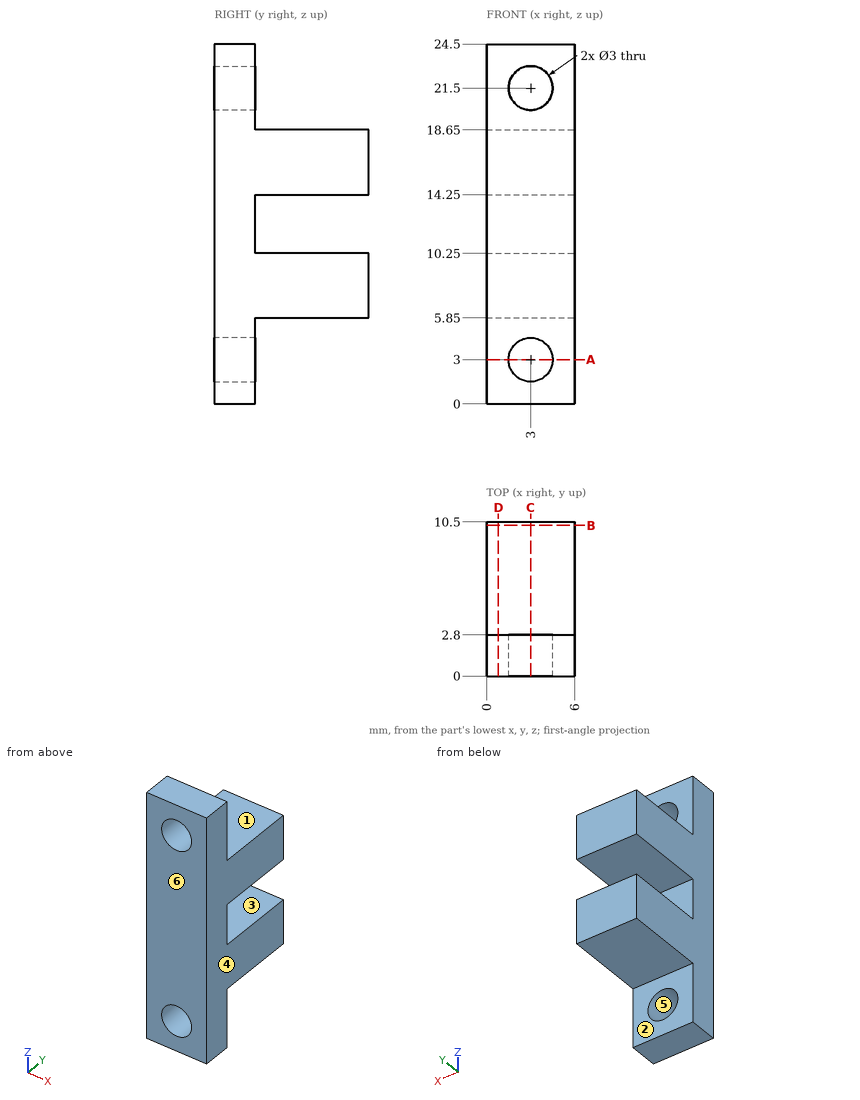
Geometry: see drawing. Coordinates: mm, zero at the bounding-box minimum. A direction names the side the tool comes from. Coordinates: 2 decimals unless noted, no trailing zeros. Order: outer loops, then holes, each group sorted by start corner. A loop starts at its lowest first (then second) coordinate and runs counter-clockwise, first axis right, second up. Notation, with made-up numbers: (6.5, 19.25) - (12.5, 19.25) arc R32 ccw to (12.5, 58.25) - close; hole circle Ø10 at (-35.5, 52). An arc over 180 degrees is marked (long way). Write each question's results on one line, items separated by ' | '.
(1) Section query B-B, the plane y = 10.25. Return the cut outline in (x, z).
Values found:
outline: (0, 5.85) - (6, 5.85) - (6, 10.25) - (0, 10.25) - close; (0, 14.25) - (6, 14.25) - (6, 18.65) - (0, 18.65) - close
(2) Section query A-A, the plane z = 3. Return the cut outline in (x, y), plus the area to 3 significant figures.
Values found:
outline: (0, 0) - (1.5, 0) - (1.5, 2.8) - (0, 2.8) - close; (4.5, 0) - (6, 0) - (6, 2.8) - (4.5, 2.8) - close | area: 8.40 mm²
(3) Line query: line 1 (Z direction, x = 2.65, y = 3.5); line 2 (X direction, y = 0.8, z = 3); line 3 (Z direction, x = 1.7, y = 2). Output: solid intervals per line, ascending. Write a range as [from, to].
Values found:
line 1: z = [5.85, 10.25], [14.25, 18.65] | line 2: x = [0, 1.5], [4.5, 6] | line 3: z = [0, 2.25], [3.75, 20.75], [22.25, 24.5]
(4) Section query C-C, the plane x = 3. Return the cut outline in (y, z).
Values found:
outline: (0, 0) - (2.8, 0) - (2.8, 1.5) - (0, 1.5) - close; (0, 4.5) - (2.8, 4.5) - (2.8, 5.85) - (10.5, 5.85) - (10.5, 10.25) - (2.8, 10.25) - (2.8, 14.25) - (10.5, 14.25) - (10.5, 18.65) - (2.8, 18.65) - (2.8, 20) - (0, 20) - close; (0, 23) - (2.8, 23) - (2.8, 24.5) - (0, 24.5) - close
(5) Mould query, pull axis X, two halves, no side actions, for the marked faces 4, 5 and 6. Classes: +X half, -X half, draft (parallel to the pull), parting line (faces both ways), or undercut.
Values found:
face 4: +X half | face 5: undercut | face 6: draft
(6) Section query D-D, the plane x = 0.8. Return the cut outline in (y, z).
Values found:
outline: (0, 0) - (2.8, 0) - (2.8, 5.85) - (10.5, 5.85) - (10.5, 10.25) - (2.8, 10.25) - (2.8, 14.25) - (10.5, 14.25) - (10.5, 18.65) - (2.8, 18.65) - (2.8, 24.5) - (0, 24.5) - close
(7) First-contact query: pin 1 Ø1.8 at (x, y) = (2.5, 7.5) entering from +Z; pin 2 Ø2 at (x, z) = (3.5, 10.5) entering from -Y; pin 3 Ø1.2 at (x, z) = (2.5, 12) entering from +Y; pin 4 Ø1.8 at (x, y) = (3.5, 6) entering from -Z. Flat tips, straight axial feed; report the tip coordinate or a pass-through.
Values found:
pin 1: stops at z = 18.65 | pin 2: stops at y = 0 | pin 3: stops at y = 2.8 | pin 4: stops at z = 5.85
(8) Set-up query: the marked faces 1, 2 and 3. Return all of +Z, -Z, +X, -X, +Y, -Y with unobstructed straight access to the full face (end or side cutting, diameter ignored); none if empty.
Values found:
face 1: +Z, +X, -X, +Y | face 2: -Z, +X, -X, +Y | face 3: +X, -X, +Y
